Geometry: final body of the model. Coordinates: model frame, mm. Face numbers are marked on the shaded views. A direction names the side the tool comes from. Give positions to 0.01 mm unless a question says otherwise; leave off trailing zeros. Loops run counter-clockwise (first coordinate to the right, second up) from the corner with the lowest first, then second, coordinate; pieces in that order, holes last. Notation, with made-up numbers: (21.25, 74.25) - (37.25, 74.25) arc R30 cw to (37.25, 106.25) - close; hole circle Ø8 at (34, 27). An arc over 180 degrees is marked (long way). Answer in a Markdown table with one row per item.
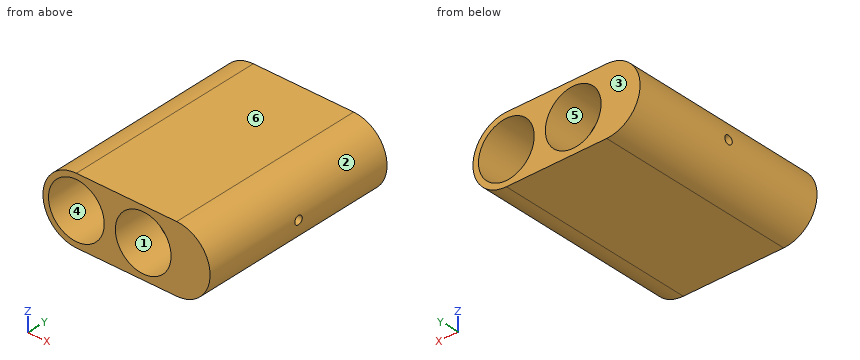
from build123d import *

# Parameters (mm, degrees)
F1_DEPTH      = 360
F2_R          = 7.5
F3_DEPTH      = 60.001
F3_DEPTH_BACK = 240.001
F4_START      = 280
F4_DEPTH      = 80
F5_DEPTH      = 80


with BuildPart() as f1:
    # F0 (on Front) → F1 (new body)
    with BuildSketch(Plane.XZ):
        with BuildLine():
            Line((180, 60), (0, 60))
            ThreePointArc((0, 60), (-60, 0), (0, -60))
            Line((0, -60), (180, -60))
            ThreePointArc((180, -60), (240, 0), (180, 60))
        make_face()
        with BuildLine():
            ThreePointArc((30, -40), (-50, 0), (30, 40))
            ThreePointArc((30, 40), (60, 50), (90, 40))
            ThreePointArc((90, 40), (120, 50), (150, 40))
            ThreePointArc((150, 40), (202.360679775, 44.72135955), (230, 0))
            ThreePointArc((230, 0), (202.360679775, -44.72135955), (150, -40))
            ThreePointArc((150, -40), (120, -50), (90, -40))
            ThreePointArc((90, -40), (60, -50), (30, -40))
        make_face(mode=Mode.SUBTRACT)
    extrude(amount=F1_DEPTH)

    # F2 (on Right) → F3 (cut, two sides)
    with BuildSketch(Plane.YZ) as f3_sk:
        with Locations((-180, 0)):
            Circle(F2_R)
    extrude(amount=-F3_DEPTH, mode=Mode.SUBTRACT)
    extrude(f3_sk.sketch, amount=F3_DEPTH_BACK, mode=Mode.SUBTRACT)

    # F0 (on Front) → F4 (join)
    with BuildSketch(Plane.XZ.offset(F4_START)):
        with BuildLine():
            ThreePointArc((30, 40), (44.72135955, 22.360679775), (50, 0))
            Line((50, 0), (60, 0))
            Line((60, 0), (70, 0))
            ThreePointArc((70, 0), (75.27864045, 22.360679775), (90, 40))
            ThreePointArc((90, 40), (60, 50), (30, 40))
        make_face()
        with BuildLine():
            Line((60, 0), (50, 0))
            ThreePointArc((50, 0), (44.72135955, -22.360679775), (30, -40))
            ThreePointArc((30, -40), (60, -50), (90, -40))
            ThreePointArc((90, -40), (75.27864045, -22.360679775), (70, 0))
            Line((70, 0), (60, 0))
        make_face()
        with BuildLine():
            ThreePointArc((230, 0), (202.360679775, 44.72135955), (150, 40))
            ThreePointArc((150, 40), (164.72135955, 22.360679775), (170, 0))
            ThreePointArc((170, 0), (164.72135955, -22.360679775), (150, -40))
            ThreePointArc((150, -40), (202.360679775, -44.72135955), (230, 0))
        make_face()
    extrude(amount=F4_DEPTH)

    # F0 (on Front) → F5 (join)
    with BuildSketch(Plane.XZ):
        with BuildLine():
            ThreePointArc((10, 0), (15.27864045, 22.360679775), (30, 40))
            ThreePointArc((30, 40), (-50, 0), (30, -40))
            ThreePointArc((30, -40), (15.27864045, -22.360679775), (10, 0))
        make_face()
        with BuildLine():
            ThreePointArc((150, 40), (120, 50), (90, 40))
            ThreePointArc((90, 40), (104.72135955, 22.360679775), (110, 0))
            Line((110, 0), (120, 0))
            Line((120, 0), (130, 0))
            ThreePointArc((130, 0), (135.27864045, 22.360679775), (150, 40))
        make_face()
        with BuildLine():
            ThreePointArc((110, 0), (104.72135955, -22.360679775), (90, -40))
            ThreePointArc((90, -40), (120, -50), (150, -40))
            ThreePointArc((150, -40), (135.27864045, -22.360679775), (130, 0))
            Line((130, 0), (120, 0))
            Line((120, 0), (110, 0))
        make_face()
    extrude(amount=F5_DEPTH)


solid = f1.part
Q1. Material intervals for line 1 along X through (y, z) = (-58, 0); line 2 along X through (y, z) = (-151.5, 0); line 3 along Z through (x, y) = (0.5, -132), sorted ascending.
Check values:
| item | result |
|---|---|
| line 1 | -60 to 10, 110 to 130, 230 to 240 |
| line 2 | -60 to -50, 230 to 240 |
| line 3 | -60 to -50, 50 to 60 |
Q2. Draft query along X for the marked faces 1, 2 and 3. Return one class per face: pulls with the +X half, pulls with the -X half, needs draft (parallel to the pull), parting line crosses it, or undercut.
Check values:
| item | result |
|---|---|
| face 1 | undercut |
| face 2 | pulls with the +X half |
| face 3 | needs draft |
Q3. Cut plane B-B (y = -265). Output: boundary loops of the cut face in (x, z).
Check values:
| item | result |
|---|---|
| outline | (0, -60) - (180, -60) arc R60 ccw to (180, 60) - (0, 60) arc R60 ccw to start; hole (30, -40) arc R50 ccw to (90, -40) arc R50 ccw to (150, -40) arc R50 ccw (long way) to (150, 40) arc R50 ccw to (90, 40) arc R50 ccw to (30, 40) arc R50 ccw (long way) to start |
Q4. Cut plane C-C (x = 161). Output: boundary loops of the cut face in (y, z).
Check values:
| item | result |
|---|---|
| outline | (-360, -60) - (0, -60) - (0, -46.25) - (-280, -46.25) - (-280, -28.62) - (-360, -28.62) - close; (-360, 28.62) - (-280, 28.62) - (-280, 46.25) - (0, 46.25) - (0, 60) - (-360, 60) - close |
Q5. Cut plane D-D (z = -23.5). Output: boundary loops of the cut face in (x, y), and give its area (4 significant figures).
Check values:
| item | result |
|---|---|
| outline | (-55.21, -360) - (-44.13, -360) - (-44.13, -80) - (15.87, -80) - (15.87, 0) - (-55.21, 0) - close; (44.13, -360) - (75.87, -360) - (75.87, -280) - (44.13, -280) - close; (104.13, -80) - (135.87, -80) - (135.87, 0) - (104.13, 0) - close; (164.13, -360) - (235.21, -360) - (235.21, 0) - (224.13, 0) - (224.13, -280) - (164.13, -280) - close |
| area | 22,650 mm² |
Q6. First-contact query: pin 1 (18 mm diameter, centred on x = 118.5, z = -24, fed in from -Y); pin 2 (12 mm diameter, centred on y = -172, z = 42, fed in from +X); pin 3 (4 mm diameter, centred on x = 187, y = -196, fed in from -Z). Flat tips, straight axial feed; report the tip coordinate or a pass-through.
Check values:
| item | result |
|---|---|
| pin 1 | y = -80 |
| pin 2 | x = 228 |
| pin 3 | z = -59.79 |
Q7. Cut plane A-A (z = 0). Output: boundary loops of the cut face in (x, y), and give its area (3 significant figures).
Check values:
| item | result |
|---|---|
| outline | (-60, -360) - (-50, -360) - (-50, -187.5) - (-60, -187.5) - close; (-60, -172.5) - (-50, -172.5) - (-50, -80) - (10, -80) - (10, 0) - (-60, 0) - close; (50, -360) - (70, -360) - (70, -280) - (50, -280) - close; (110, -80) - (130, -80) - (130, 0) - (110, 0) - close; (170, -360) - (240, -360) - (240, -187.5) - (230, -187.5) - (230, -280) - (170, -280) - close; (230, -172.5) - (240, -172.5) - (240, 0) - (230, 0) - close |
| area | 19,700 mm² |
Q8. Reachability of the marked faces 4, 5 and 6 from +Z, -Z, +X, -X, +Y, -Y: full face, straight path, thin tool, end or side. Return the list, or none.
Check values:
| item | result |
|---|---|
| face 4 | -Y |
| face 5 | +Y |
| face 6 | +Z, +X, -X, +Y, -Y |
